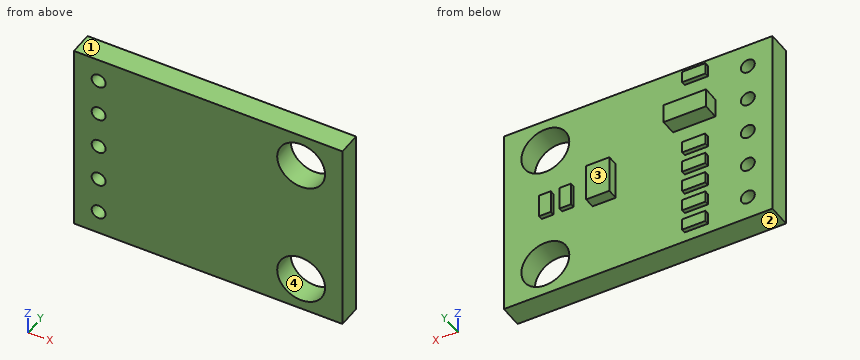
from build123d import *

# Parameters (mm, degrees)
SKETCH2_W               = 18.5
SKETCH2_H               = 13.4
BOSS_EXTRUDE1_DEPTH     = 1.6
CUT_EXTRUDE1_DEPTH      = 12.533104526
CUT_EXTRUDE1_DEPTH_BACK = 12.533104526
SKETCH3_R               = 0.48
SKETCH3_R_2             = 1.65
SKETCH6_W               = 1.6
SKETCH6_H               = 0.8
SKETCH6_W_2             = 0.8
SKETCH6_H_2             = 1.6
BOSS_EXTRUDE2_DEPTH     = 0.3
SKETCH7_W               = 2.92
SKETCH7_H               = 1.32
BOSS_EXTRUDE3_DEPTH     = 1.1
SKETCH8_W               = 1.6
SKETCH8_H               = 2.6
BOSS_EXTRUDE4_DEPTH     = 0.75


with BuildPart() as part:
    # Sketch2 → Boss-Extrude1 (new body)
    with BuildSketch(Plane(origin=(0, 0, 0), x_dir=(1, 0, 0), z_dir=(0, 1, 0))):
        Rectangle(SKETCH2_W, SKETCH2_H)
    extrude(amount=BOSS_EXTRUDE1_DEPTH)

    # Sketch3 → Cut-Extrude1 (cut, two sides: drawn at the far end of the back side and taken through both)
    with BuildSketch(Plane(origin=(0, 1.6, 0), x_dir=(1, 0, 0), z_dir=(0, 1, 0)).offset(-CUT_EXTRUDE1_DEPTH_BACK)):
        with Locations(Location((-7.55, 5.08, 0), (0, 0, 270))):
            Circle(SKETCH3_R)
        with Locations(Location((-7.55, 2.54, 0), (0, 0, 270))):
            Circle(SKETCH3_R)
        with Locations(Location((-7.55, 0, 0), (0, 0, 270))):
            Circle(SKETCH3_R)
        with Locations(Location((-7.55, -2.54, 0), (0, 0, 270))):
            Circle(SKETCH3_R)
        with Locations(Location((-7.55, -5.08, 0), (0, 0, 270))):
            Circle(SKETCH3_R)
        with Locations(Location((6.4, 4.4, 0), (0, 0, 270))):
            Circle(SKETCH3_R_2)
        with Locations(Location((6.4, -4.4, 0), (0, 0, 270))):
            Circle(SKETCH3_R_2)
    extrude(amount=CUT_EXTRUDE1_DEPTH + CUT_EXTRUDE1_DEPTH_BACK, mode=Mode.SUBTRACT)

    # Sketch6 → Boss-Extrude2 (add)
    with BuildSketch(Plane(origin=(0, 1.6, 0), x_dir=(1, 0, 0), z_dir=(0, 1, 0))):
        with Locations((-4, 5.6)):
            Rectangle(SKETCH6_W, SKETCH6_H)
        with Locations((-4, 4.1)):
            Rectangle(SKETCH6_W, SKETCH6_H)
        with Locations((-4, 2.6)):
            Rectangle(SKETCH6_W, SKETCH6_H)
        with Locations((-4, 1.1)):
            Rectangle(SKETCH6_W, SKETCH6_H)
        with Locations((-4, -0.4)):
            Rectangle(SKETCH6_W, SKETCH6_H)
        with Locations((-4, -5.85)):
            Rectangle(SKETCH6_W, SKETCH6_H)
        with Locations((6.25, 0)):
            Rectangle(SKETCH6_W_2, SKETCH6_H_2)
        with Locations((4.85, 0)):
            Rectangle(SKETCH6_W_2, SKETCH6_H_2)
    extrude(amount=BOSS_EXTRUDE2_DEPTH)

    # Sketch7 → Boss-Extrude3 (add)
    with BuildSketch(Plane(origin=(0, 1.6, 0), x_dir=(1, 0, 0), z_dir=(0, 1, 0))):
        with Locations((-3.85, -2.77)):
            Rectangle(SKETCH7_W, SKETCH7_H)
    extrude(amount=BOSS_EXTRUDE3_DEPTH)

    # Sketch8 → Boss-Extrude4 (add)
    with BuildSketch(Plane(origin=(0, 1.6, 0), x_dir=(1, 0, 0), z_dir=(0, 1, 0))):
        with Locations((2.35, 0)):
            Rectangle(SKETCH8_W, SKETCH8_H)
    extrude(amount=BOSS_EXTRUDE4_DEPTH)


solid = part.part
Here's how the part is built. I have some questions about the finished solid (model axes, mm). Face numbers are marked on the shaded views. Coordinates: 2 decimals unless noted, no trailing zeros. Order: outer loops, then holes, each group sorted by start corner. A loop starts at its lowest first (then second) coordinate and runs counter-clockwise, first axis right, second up. Notation, with made-up numbers: (50, 41) -> (85, 41) arc R21 ccw to (85, 74) -> close; hole circle Ø8 at (-9, 77.5). An arc over 180 degrees is marked (long way). Answer in a Markdown table with one row per item.
(1) Will these pins go through, and if not, where does the flat tip stop? pin 1 Ø2 at (x, z) = (3, -3) entering from +Y; pin 2 Ø1.8 at (x, z) = (2.5, -0.5) entering from +Y.
Answer key:
| item | result |
|---|---|
| pin 1 | y = 1.6 |
| pin 2 | y = 2.35 |
(2) I want a section at C-C on z = 2.54. List the corners of the cut face in (x, y) for me.
Answer key:
| item | result |
|---|---|
| outline | (-9.25, 0) -> (-8.03, 0) -> (-8.03, 1.6) -> (-9.25, 1.6) -> close; (-7.07, 0) -> (9.25, 0) -> (9.25, 1.6) -> (-2.39, 1.6) -> (-2.39, 2.7) -> (-5.31, 2.7) -> (-5.31, 1.6) -> (-7.07, 1.6) -> close |
(3) Thinking about a two-plate mould opening in Z: for the marked faces 1, 2, 3 and 4, which applies, +Z half, -Z half, draft (parallel to the pull), parting line (faces both ways), or undercut?
Answer key:
| item | result |
|---|---|
| face 1 | +Z half |
| face 2 | -Z half |
| face 3 | draft |
| face 4 | undercut |
(4) I want a section at D-D on x = 6.4. List the corners of the cut face in (y, z) for me.
Answer key:
| item | result |
|---|---|
| outline | (0, -6.7) -> (1.6, -6.7) -> (1.6, -6.05) -> (0, -6.05) -> close; (0, -2.75) -> (1.6, -2.75) -> (1.6, -0.8) -> (1.9, -0.8) -> (1.9, 0.8) -> (1.6, 0.8) -> (1.6, 2.75) -> (0, 2.75) -> close; (0, 6.05) -> (1.6, 6.05) -> (1.6, 6.7) -> (0, 6.7) -> close |
(5) I want a section at B-B on y = 0.3. List the corners of the cut face in (x, z) for me, then the cut area to 3 significant figures.
Answer key:
| item | result |
|---|---|
| outline | (-9.25, -6.7) -> (9.25, -6.7) -> (9.25, 6.7) -> (-9.25, 6.7) -> close; hole circle Ø0.96 at (-7.55, -5.08); hole circle Ø0.96 at (-7.55, -2.54); hole circle Ø0.96 at (-7.55, 0); hole circle Ø0.96 at (-7.55, 2.54); hole circle Ø0.96 at (-7.55, 5.08); hole circle Ø3.3 at (6.4, -4.4); hole circle Ø3.3 at (6.4, 4.4) |
| area | 227 mm^2 |
(6) Please list where these lines run through material, in increasing order: probe 1 along Z at (x, y) = (-7.55, 0.35); probe 2 along Z at (x, y) = (6.5, 1.25); probe 3 along Z at (x, y) = (5.25, 0.15).
Answer key:
| item | result |
|---|---|
| probe 1 | -6.7 to -5.56, -4.6 to -3.02, -2.06 to -0.48, 0.48 to 2.06, 3.02 to 4.6, 5.56 to 6.7 |
| probe 2 | -6.7 to -6.05, -2.75 to 2.75, 6.05 to 6.7 |
| probe 3 | -6.7 to -5.58, -3.22 to 3.22, 5.58 to 6.7 |
(7) I want a section at A-A on x = -7.55. List the corners of the cut face in (y, z) for me.
Answer key:
| item | result |
|---|---|
| outline | (0, -6.7) -> (1.6, -6.7) -> (1.6, -5.56) -> (0, -5.56) -> close; (0, -4.6) -> (1.6, -4.6) -> (1.6, -3.02) -> (0, -3.02) -> close; (0, -2.06) -> (1.6, -2.06) -> (1.6, -0.48) -> (0, -0.48) -> close; (0, 0.48) -> (1.6, 0.48) -> (1.6, 2.06) -> (0, 2.06) -> close; (0, 3.02) -> (1.6, 3.02) -> (1.6, 4.6) -> (0, 4.6) -> close; (0, 5.56) -> (1.6, 5.56) -> (1.6, 6.7) -> (0, 6.7) -> close |
